Can you work these out from the drawing? Everything is in mm from the part's minimum corner. Give positions to 0.01 mm unless a question says otherwise; leave off trailing zeros. Loops run counter-clockwise (first coordinate to the right, second up) from the corner with the lowest first, then second, coordinate; pieces in that order, holes last. Notation, with made-up numbers: (8, 53) - (24, 53) arc R15 ccw to (24, 57) - close; hole circle Ø10 at (17.5, -10.5). An arc over 180 degrees is marked (long way). Answer in a Markdown table with one row per item. Add a question column.
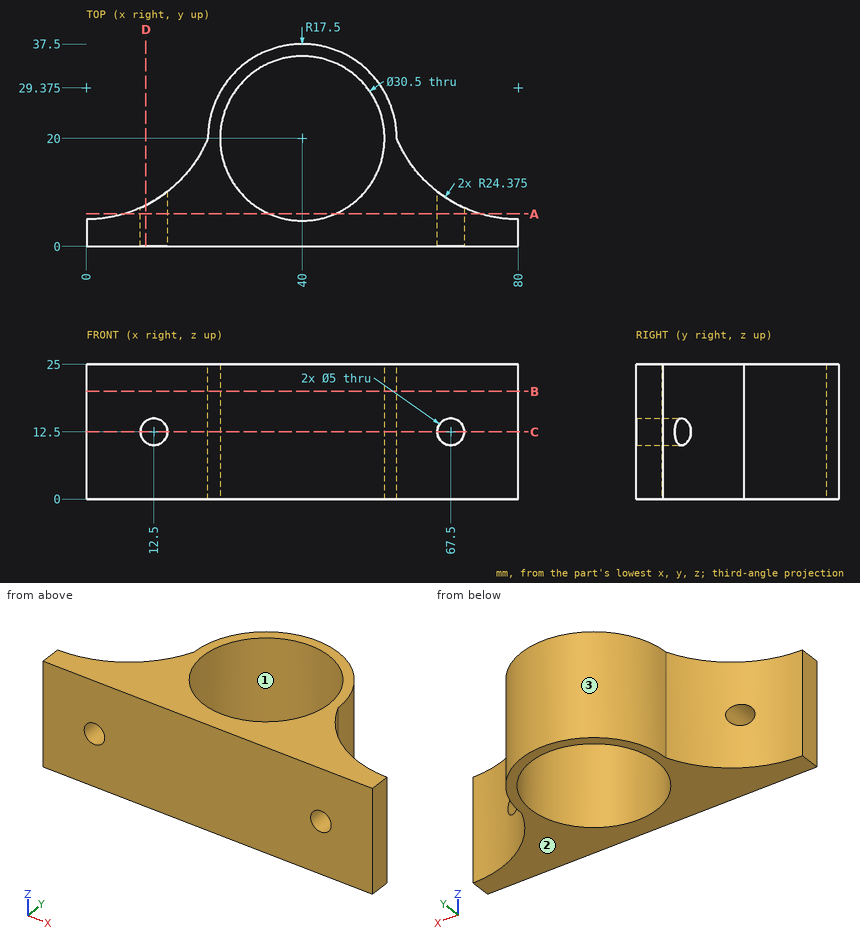
(1) We'd pull the mould along X, two halves only. Please class the marked faces 1, 2 and 3: pulls with the +X half, pulls with the -X half, needs draft (parallel to the pull), parting line crosses it, or undercut.
(2) I want a section at B-B on z = 20. Please give me the cut outline in (x, y) (3 decimals), then the cut area to 3 significant figures.
(3) I want a section at D-D on x = 11. Please give me the cut outline in (y, z).
(4) For pin 1 Ø3 at (x, z) = (16.5, 20.5) entering from +Y; pin 2 Ø10 at (x, z) = (46.5, 19.5) entering from +Y; pin 3 Ø10 at (y, z) = (13.5, 17) entering from -X; pin 4 Ø6 at (x, z) = (12.5, 12.5) entering from -Y, each with a flat end and sliding along its axis, tell me the tip position at first contact or that it passes through.
(5) I want a section at A-A on y = 6. Please give me the cut outline in (x, z), then the cut area to 3 significant figures.
(6) Please list where these lines run through material, in increasing order: line 1 (Y direction, x = 40, z = 16.25); line 2 (X direction, y = 4, z = 12); line 3 (X direction, y = 8, z = 12).
(7) I want a section at C-C on z = 12.5. Please give me the cut outline in (x, y) (3 decimals).
Reported:
| question | item | result |
|---|---|---|
| 1 | face 1 | undercut |
| 1 | face 2 | needs draft |
| 1 | face 3 | parting line crosses it |
| 2 | outline | (0, 0) - (80, 0) - (80, 5) arc R24.375 cw to (57.5, 20) arc R17.5 ccw to (22.5, 20) arc R24.375 cw to (0, 5) - close; hole circle Ø30.5 at (40, 20) |
| 2 | area | 863 mm² |
| 3 | outline | (0, 0) - (7.62, 0) - (7.62, 10.5) - (0, 10.5) - close; (0, 14.5) - (7.62, 14.5) - (7.62, 25) - (0, 25) - close |
| 4 | pin 1 | y = 12.94 |
| 4 | pin 2 | y = 37.44 |
| 4 | pin 3 | x = 12.58 |
| 4 | pin 4 | y = 0 |
| 5 | outline | (6.91, 0) - (33.95, 0) - (33.95, 25) - (6.91, 25) - close; (46.05, 0) - (73.09, 0) - (73.09, 25) - (46.05, 25) - close; hole circle Ø5 at (12.5, 12.5); hole circle Ø5 at (67.5, 12.5) |
| 5 | area | 1,310 mm² |
| 6 | line 1 | 0 to 4.75, 35.25 to 37.5 |
| 6 | line 2 | 0 to 10.05, 14.95 to 65.05, 69.95 to 80 |
| 6 | line 3 | 14.95 to 30.59, 49.41 to 65.05 |
| 7 | outline | (0, 0) - (10, 0) - (10, 7.146) arc R24.375 cw to (0, 5) - close; (15, 0) - (65, 0) - (65, 10.162) arc R24.375 cw to (57.5, 20) arc R17.5 ccw to (22.5, 20) arc R24.375 cw to (15, 10.162) - close; (70, 0) - (80, 0) - (80, 5) arc R24.375 cw to (70, 7.146) - close; hole circle Ø30.5 at (40, 20) |
